from build123d import *

# Parameters (mm, degrees)
BOSS_EXTRUDE1_DEPTH        = 6
F_3_9_3_9_DIAMETER_HOLE1_D = 3.9


with BuildPart() as part:
    # Sketch1 → Boss-Extrude1 (new body)
    with BuildSketch(Plane.XY.offset(6)):
        with BuildLine():
            Line((47.5, 4.5), (-47.5, 4.5))
            ThreePointArc((-47.5, 4.5), (-52, 0), (-47.5, -4.5))
            Line((-47.5, -4.5), (47.5, -4.5))
            ThreePointArc((47.5, -4.5), (52, 0), (47.5, 4.5))
        make_face()
    extrude(amount=-BOSS_EXTRUDE1_DEPTH)

    # Ø3.9 (3.9) Diameter Hole1 (through all)
    with Locations(Plane(origin=(0, 0, 0), x_dir=(-1, 0, 0), z_dir=(0, 0, -1))):
        with Locations((47.5, 0), (-47.5, 0)):
            Hole(F_3_9_3_9_DIAMETER_HOLE1_D / 2)

    # Sketch4 → CSK for M2.5 Flat Head Machine Screw1 (revolve, cut)
    with BuildSketch(Plane.YZ):
        Polygon((0, 0), (0, 6), (1.5, 6), (1.5, 4), (2.5, 3), (2.5, 0), align=None)
    revolve(axis=Axis((0, 0, -6.35), (0, 0, 1)), mode=Mode.SUBTRACT)


solid = part.part
Design review of the part built by this model. Coordinates are the model's own, in mm. A direction names the side the tool comes from. Give positions to 0.01 mm unless a question says otherwise; leave off trailing zeros. Order: outer loops, then holes, each group sorted by start corner. A loop starts at its lowest first (then second) coordinate and runs counter-clockwise, first axis right, second up.
1. For pin 1 Ø1 at (y, z) = (3, 2.5) entering from -X; pin 2 Ø2.5 at (x, y) = (0, 0) entering from -Z, all flat-tipped, find the tip position at first contact; note any pin that passes through.
Solution:
pin 1: stops at x = -51.24
pin 2: passes through
2. Add section A-A, the plane y = 0. State the section outline as (x, z) points, then the cut area to 3 significant figures.
Solution:
outline: (-52, 0) - (-49.45, 0) - (-49.45, 6) - (-52, 6) - close; (-45.55, 0) - (-2.5, 0) - (-2.5, 3) - (-1.5, 4) - (-1.5, 6) - (-45.55, 6) - close; (1.5, 4) - (2.5, 3) - (2.5, 0) - (45.55, 0) - (45.55, 6) - (1.5, 6) - close; (49.45, 0) - (52, 0) - (52, 6) - (49.45, 6) - close
area: 552 mm2
3. Add section C-C, the plane z = 5. State the section outline as (x, y) points.
Solution:
outline: (-47.5, -4.5) - (47.5, -4.5) arc R4.5 ccw to (47.5, 4.5) - (-47.5, 4.5) arc R4.5 ccw to start; hole circle Ø3.9 at (-47.5, 0); hole circle Ø3 at (0, 0); hole circle Ø3.9 at (47.5, 0)
4. Mouldability with a two-part tool opening along Y and no side actions: class faces 3 (the cylindrical face through (-45.7, -0.75, 3.04)), 4 (the flat face through (-1, -3, 0)), 5 (the cylindrical face through (52, 0, 3)) as +Y half, -Y half, draft (parallel to the pull), parting line (faces both ways), or undercut.
Solution:
face 3: undercut
face 4: draft
face 5: parting line
5. To check wall thickness, follow L1, parallel to Y at x = 47.5, z = 4.75; L2, parallel to Y at x = 0, z = 2.15; L3, parallel to X at y = 0.5, z = 1.85. State the ranges of each line that lie inside material, in increasing order.
Solution:
L1: y = -4.5 to -1.95, 1.95 to 4.5
L2: y = -4.5 to -2.5, 2.5 to 4.5
L3: x = -51.97 to -49.38, -45.62 to -2.45, 2.45 to 45.62, 49.38 to 51.97
6. Tool access review of faces 1 (the cylindrical face through (-52, 0, 3)), 2 (the cylindrical face through (2.44, -0.54, 1.48)): name each direction out of +Z, -Z, +X, -X, +Y, -Y from which nothing blocks a thin tool from reaching the whole face with its end or side.
Solution:
face 1: +Z, -Z, -X
face 2: -Z
7. Add section B-B, the plane x = 0. State the section outline as (y, z) points, then the cut area to 3 significant figures.
Solution:
outline: (-4.5, 0) - (-2.5, 0) - (-2.5, 3) - (-1.5, 4) - (-1.5, 6) - (-4.5, 6) - close; (1.5, 4) - (2.5, 3) - (2.5, 0) - (4.5, 0) - (4.5, 6) - (1.5, 6) - close
area: 29.0 mm2
